The drawing under review shows one solid part. Ordinate dimensions are in mm from its lowest x, y, z. A direction names the side the tool comes from. Round coordinates to 2 decimals unless told otherwise and drop trailing zeros. Write each loop counter-clockwise with the first axis right and the second up, starting at its lowest first coordinate (ties: lowest second). Pieces come first, ordered by that corner, then holes. Notation, with made-up numbers: (27.5, -8.5) - (31.5, -8.5) arc R26 cw to (31.5, 23.5) - close; hole circle Ø4 at (82.5, -9.75). An arc over 180 degrees is marked (long way). One line per question, with ' | ' between items. Start each with the question number.
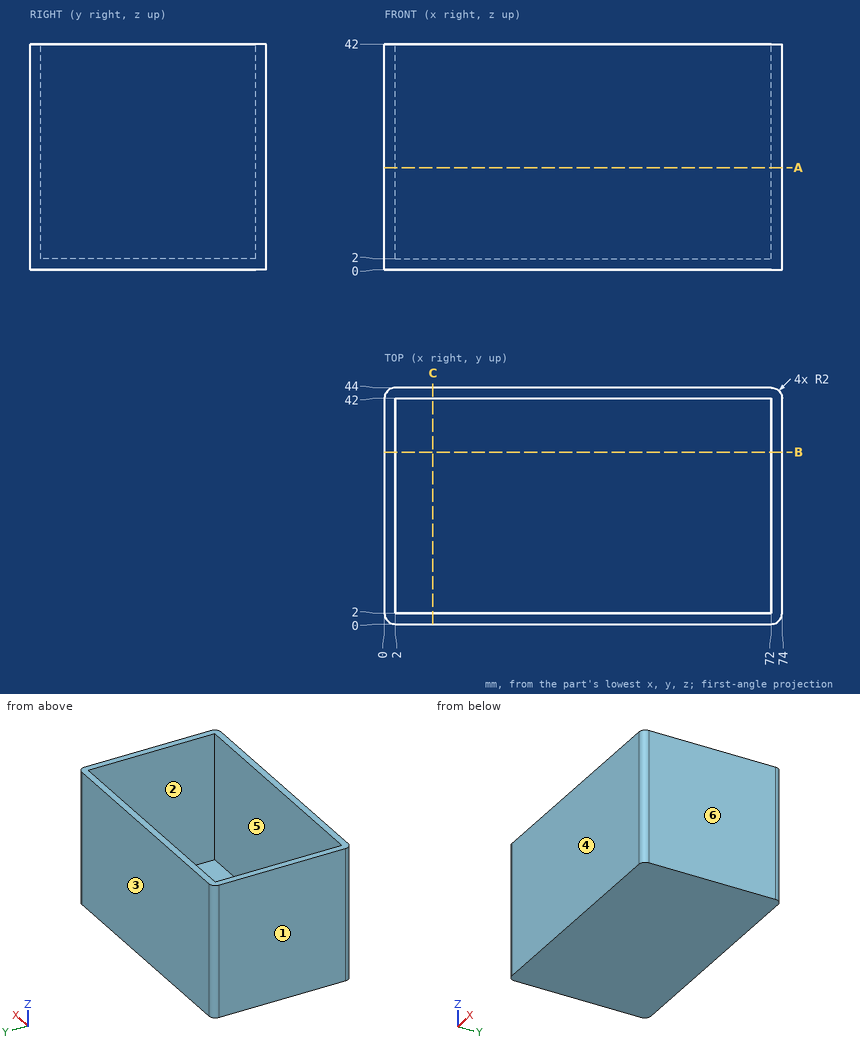
1. Add section B-B, the plane y = 32. Write out the cut boundary in (x, z), then the cut area to 3 significant figures.
2. Clearance check with flat-ended pins moving along their axes: P1, Ø8, axis at x = 28, y = 9.5, coming from the +Z side; P2, Ø1, axis at x = 10, y = 6.5, coming from the -Z side. State where each tip first meets the part, or that it passes through.
3. Add section C-C, the plane x = 9. Write out the cut boundary in (y, z).
4. Add section A-A, the plane z = 19. Write out the cut boundary in (x, y).
5. Wall thickness on line 1 along Y through (x, z) = (13, 24.5); line 2 along X through (y, z) = (18, 29.5); line 3 along Z through (x, y) = (14, 13): over which ranges is each line inside the solid? List them lowest first. Write a range as [from, to].
6. The part is to be moulded in two halves that separate along Y. For the marked faces 1, 2, 3 and 4, say which applies: pulls with the +Y half, pulls with the -Y half, needs draft (parallel to the pull), parting line crosses it, or undercut.
7. Machinability: for the marked faces 5 and 6, which of the approach directions +Z, -Z, +X, -X, +Y, -Y give a long, thin tool a straight path to every point of the face, cutting with its end or side? Answer none if there is none.
Geometry check:
1) outline: (0, 0) - (74, 0) - (74, 42) - (72, 42) - (72, 2) - (2, 2) - (2, 42) - (0, 42) - close | area: 308 mm2
2) P1: stops at z = 2 | P2: stops at z = 0
3) outline: (0, 0) - (44, 0) - (44, 42) - (42, 42) - (42, 2) - (2, 2) - (2, 42) - (0, 42) - close
4) outline: (0, 2) arc R2 ccw to (2, 0) - (72, 0) arc R2 ccw to (74, 2) - (74, 42) arc R2 ccw to (72, 44) - (2, 44) arc R2 ccw to (0, 42) - close; hole (2, 2) - (72, 2) - (72, 42) - (2, 42) - close
5) line 1: y = [0, 2], [42, 44] | line 2: x = [0, 2], [72, 74] | line 3: z = [0, 2]
6) face 1: needs draft | face 2: undercut | face 3: pulls with the +Y half | face 4: pulls with the -Y half
7) face 5: +Z | face 6: +Z, -Z, +X, +Y, -Y
